Input: part model. Units: mm. Frame: model coordinates. Face numbers are marked on the shaded views. A direction names the side the tool comes from. Give positions to 0.01 mm unless a question says otherwise; leave off trailing zeros. Write each loop counter-clockwise with the first axis right and the second up, starting at its lowest first coordinate (ties: lowest second). Pieces come first, ordered by that corner, then holes.
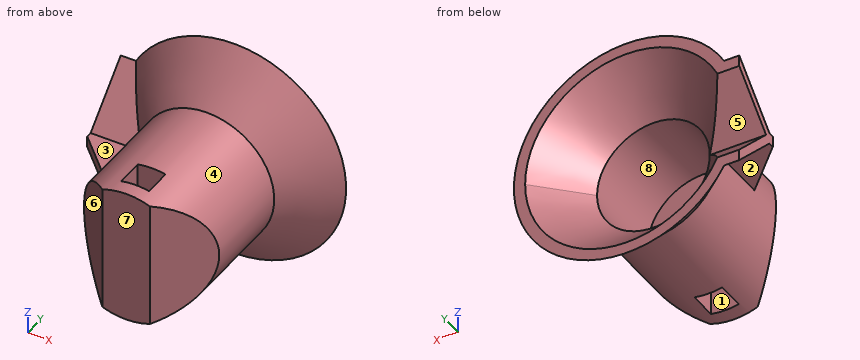
```python
from build123d import *

# Parameters (mm, degrees)
SKETCH1_R               = 9
BOSS_EXTRUDE1_DEPTH     = 18
CUT_EXTRUDE1_DEPTH      = 23.045407685
CUT_EXTRUDE1_DEPTH_BACK = 23.045407685
SKETCH2_W               = 3.7
SKETCH2_H               = 3.7
CUT_EXTRUDE2_START      = -11.3
SKETCH3_R               = 7.5
CUT_EXTRUDE2_DEPTH      = 11.3
CUT_EXTRUDE3_DEPTH      = 33.031234756
BOSS_EXTRUDE2_REACH     = 43.243
BOSS_EXTRUDE4_DEPTH     = 0.75


with BuildPart() as part:
    # Sketch1 → Boss-Extrude1 (new body)
    with BuildSketch(Plane(origin=(0, 0, 0), x_dir=(1, 0, 0), z_dir=(0, 1, 0))):
        with Locations(Location((0, 0, 0), (0, 0, 270))):
            Circle(SKETCH1_R)
    extrude(amount=BOSS_EXTRUDE1_DEPTH)

    # Sketch2 → Cut-Extrude1 (cut, two sides: drawn at the far end of the back side and taken through both)
    with BuildSketch(Plane.XY.offset(-CUT_EXTRUDE1_DEPTH_BACK)):
        Polygon((-9, 5.7), (-3.175, 0), (-9, 0), align=None)
        Polygon((3.175, 0), (9, 5.7), (9, 0), align=None)
        with Locations((0, 3.85)):
            Rectangle(SKETCH2_W, SKETCH2_H)
    extrude(amount=CUT_EXTRUDE1_DEPTH + CUT_EXTRUDE1_DEPTH_BACK, mode=Mode.SUBTRACT)

    # Sketch3 → Cut-Extrude2 (cut)
    with BuildSketch(Plane(origin=(0, 18, 0), x_dir=(1, 0, 0), z_dir=(0, 1, 0)).offset(CUT_EXTRUDE2_START)):
        with Locations(Location((0, 0, 0), (0, 0, 270))):
            Circle(SKETCH3_R)
    extrude(amount=CUT_EXTRUDE2_DEPTH, mode=Mode.SUBTRACT)

    # Sketch4 → Revolve1 (revolve)
    with BuildSketch(Plane.XY):
        Polygon((9, 18), (15, 24), (13.5, 24), (7.5, 18), align=None)
    revolve(axis=Axis((0, -14.513203436, 0), (0, 1, 0)))

    # Sketch5 → Cut-Extrude3 (cut, through all)
    with BuildSketch(Plane(origin=(0, 0, 0), x_dir=(0, 0, -1), z_dir=(1, 0, 0))):
        Polygon((0, 18), (-6, 24), (6, 24), align=None)
    extrude(amount=-CUT_EXTRUDE3_DEPTH, mode=Mode.SUBTRACT)

    # Sketch6 → Boss-Extrude2 (add, up to next)
    with BuildSketch(Plane(origin=(-15, 0, 0), x_dir=(0, 0, -1), z_dir=(1, 0, 0)), mode=Mode.PRIVATE) as boss_extrude2_sk1:
        Polygon((6, 24), (0, 18), (-6, 24), (-7.5, 24), (0, 16.5), (7.5, 24), align=None)
    boss_extrude2_tool1 = extrude(boss_extrude2_sk1.sketch, amount=BOSS_EXTRUDE2_REACH, mode=Mode.PRIVATE) - part.part
    add(boss_extrude2_tool1.solids().sort_by_distance((-15, 20.881415, -3.118585))[0])

    # Sketch7 → Boss-Extrude4 (add, symmetric)
    with BuildSketch(Plane.XY):
        Polygon((-15, 18), (-15, 16.5), (-7.5, 9), (-7.5, 18), align=None)
    extrude(amount=BOSS_EXTRUDE4_DEPTH, both=True)


solid = part.part
```
Q1. Pin query (flat end, axial travel): pin 1 (5 mm diameter, centred on x = 6.5, y = 5, fed in from +Z); pin 2 (5 mm diameter, centred on y = 6, z = 10.5, fed in from +X); pin 3 (1.5 mm diameter, centred on x = -6.5, z = -0.5, fed in from +Y). Return the tip coordinate at first contact, or that it passes through.
Q2. Mould query, pull axis X, two halves, no side actions, for the marked faces 6, 7 and 8. Classes: +X half, -X half, draft (parallel to the pull), parting line (faces both ways), or undercut.
Q3. Access query for the marked faces 1, 2, 3, 4 and 5. Directions: +Z, -Z, +X, -X, +Y, -Y. A direction counts if a zero-diameter tool reaches every point of the face in a straight line with its end or side. Return the directions, or none.
Q4. Section B-B, the plane y = 12.25. Return the cut outline in (x, z).
Q5. Material intervals for line 1 along X through (y, z) = (9.5, 0); line 2 along Y through (x, z) = (-1, -4), sorted ascending.
Q6. Section A-A, the plane x = 0. Return the cut outline in (y, z).
Solutions:
1. pin 1: stops at z = 8.06
1. pin 2: stops at x = 4.12
1. pin 3: stops at y = 6.7
2. face 6: -X half
2. face 7: draft
2. face 8: undercut
3. face 1: +Z, -Z
3. face 2: -Z, -X, -Y
3. face 3: +Z, -X, -Y
3. face 4: -Y
3. face 5: -X, +Y
4. outline: (-10.75, -0.75) - (-8.97, -0.75) arc R9 ccw (long way) to (-8.97, 0.75) - (-10.75, 0.75) - close; hole circle Ø15 at (0, 0)
5. line 1: x = -9 to -7.5, 7.5 to 9
5. line 2: y = 0 to 2, 5.7 to 6.7
6. outline: (0, -9) - (2, -9) - (2, 9) - (0, 9) - close; (5.7, -9) - (18, -9) - (24, -15) - (24, -13.5) - (18, -7.5) - (6.7, -7.5) - (6.7, 7.5) - (18, 7.5) - (24, 13.5) - (24, 15) - (18, 9) - (5.7, 9) - close
